Can you work these out from the drawing? Everything is in mm from the part's minimum corner. Give positions to 0.01 mm unless a question says otherwise; leave off trailing zeros. Order: outer loops, then holes, each group sorted by start corner. A loop starts at its lowest first (then second) coordinate and runs counter-clockwise, first axis right, second up. Notation, with made-up numbers: (64.5, -24) -> (70.5, -24) arc R24 cw to (70.5, 13) -> close; hole circle Ø1 at (33.25, 60). An arc over 180 degrees is marked (long way). Answer as CSV lines item,"result". Start each with the question number.
(1) I want a section at A-A (z = 55). Please give me the cut outline in (x, y).
(2) I want a section at D-D (z = 44.5). Please give me the cut outline in (x, y).
(3) I need wall thicknesses on L1, parallel to Y at x = 4, z = 55; L2, parallel to Z at x = 4.65, y = 94; L3, parallel to Y at x = 4.5, z = 65. Which ranges of each line are inside material? Lowest first, please.
(4) Will this pin go through, and if not, where does the flat tip stop? pin 1 Ø2 at (x, y) = (3.5, 90.5) entering from -Z.
(5) I want a section at C-C (x = 4.25). Please give me the cut outline in (y, z).
(6) I want a section at B-B (y = 95). Please give me the cut outline in (x, z).
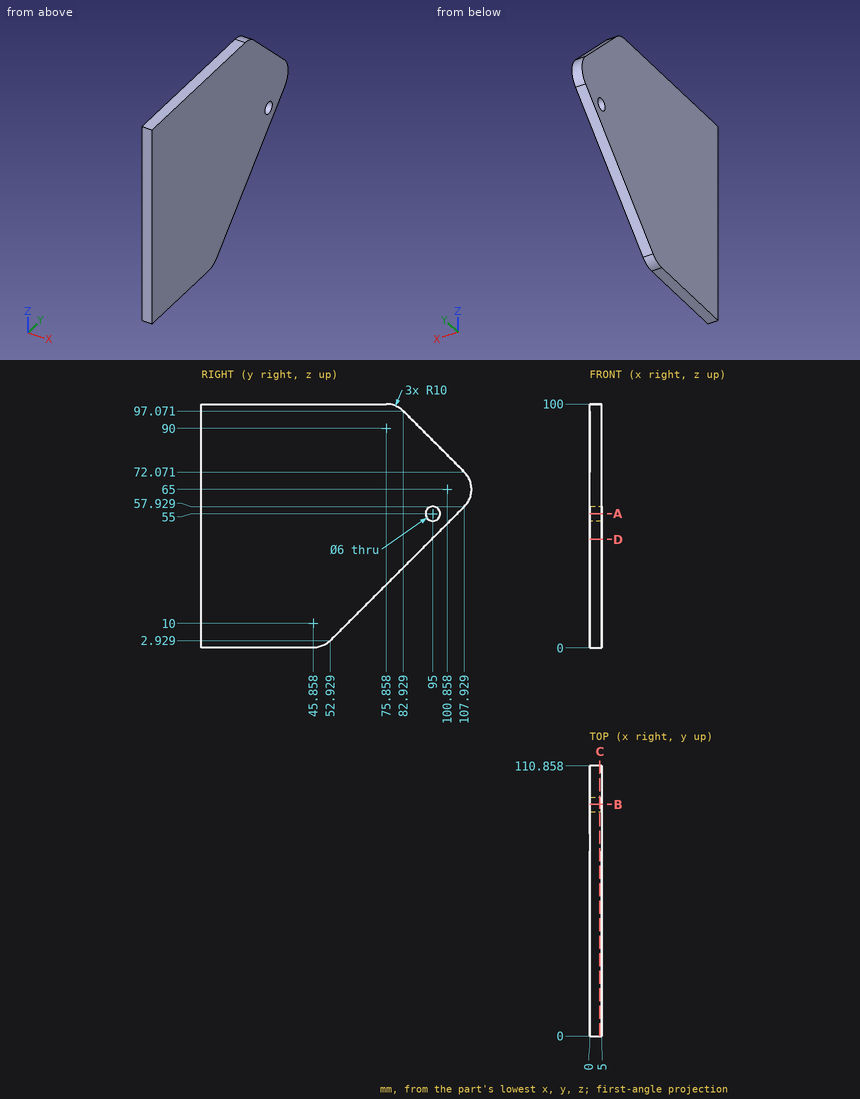
Final values:
1,outline,"(0, 0) -> (5, 0) -> (5, 92) -> (0, 92) -> close; (0, 98) -> (5, 98) -> (5, 105) -> (0, 105) -> close"
2,outline,"(0, 0) -> (5, 0) -> (5, 94.5) -> (0, 94.5) -> close"
3,L1,"0 to 92, 98 to 105"
3,L2,"44 to 52.17, 57.83 to 86"
3,L3,"0 to 110.86"
4,pin 1,"z = 39.5"
5,outline,"(0, 0) -> (45.86, 0) arc R10 ccw to (52.93, 2.93) -> (107.93, 57.93) arc R10 ccw to (107.93, 72.07) -> (82.93, 97.07) arc R10 ccw to (75.86, 100) -> (0, 100) -> close; hole circle Ø6 at (95, 55)"
6,outline,"(0, 45) -> (5, 45) -> (5, 52) -> (0, 52) -> close; (0, 58) -> (5, 58) -> (5, 85) -> (0, 85) -> close"
